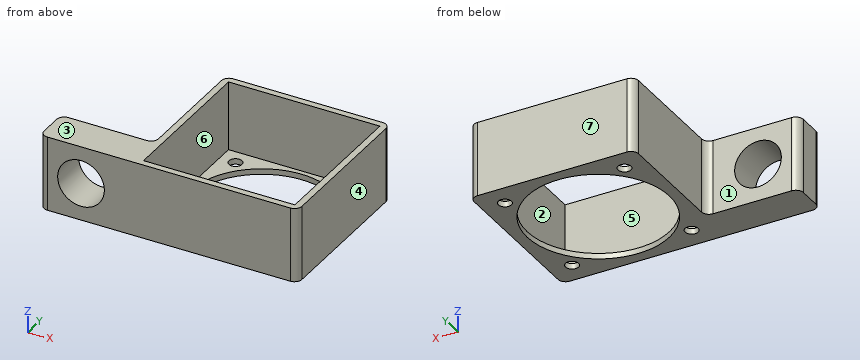
from build123d import *

# Parameters (mm, degrees)
F0_W     = 44
F0_H     = 44
F0_W_2   = 40.5
F0_H_2   = 40.5
F1_DEPTH = 20
F0_R     = 1.75
F0_R_2   = 19
F2_DEPTH = 1.5
F3_W     = 10
F3_H     = 20
F4_DEPTH = 25
F5_R     = 6.25
F6_DEPTH = 10
F7_R     = 2


with BuildPart() as f1:
    # F0 (on Top) → F1 (new body)
    with BuildSketch(Plane.XY):
        Rectangle(F0_W, F0_H)
        Rectangle(F0_W_2, F0_H_2, mode=Mode.SUBTRACT)
    extrude(amount=F1_DEPTH)

    # F0 (on Top) → F2 (join)
    with BuildSketch(Plane.XY):
        Rectangle(F0_W_2, F0_H_2)
        with Locations((-16, -16)):
            Circle(F0_R, mode=Mode.SUBTRACT)
        with Locations((16, -16)):
            Circle(F0_R, mode=Mode.SUBTRACT)
        with Locations((-16, 16)):
            Circle(F0_R, mode=Mode.SUBTRACT)
        Circle(F0_R_2, mode=Mode.SUBTRACT)
        with Locations((16, 16)):
            Circle(F0_R, mode=Mode.SUBTRACT)
    extrude(amount=F2_DEPTH)

    # F3 (on face) → F4 (join)
    with BuildSketch(Plane(origin=(-22, 0, 0), x_dir=(0, -1, 0), z_dir=(-1, 0, 0))):
        with Locations((17, 10)):
            Rectangle(F3_W, F3_H)
    extrude(amount=F4_DEPTH)

    # F5 (on face) → F6 (cut)
    with BuildSketch(Plane(origin=(0, -12, 0), x_dir=(-1, 0, 0), z_dir=(0, 1, 0))):
        with Locations((36, 10)):
            Circle(F5_R)
    extrude(amount=-F6_DEPTH, mode=Mode.SUBTRACT)

    # F7
    f7_edges = [f1.edges().sort_by_distance(p)[0] for p in [
        (-22, -12, 10),
        (-22, 22, 10),
        (22, 22, 10),
        (22, -22, 10),
        (-47, -12, 10),
        (-47, -22, 10),
    ]]
    fillet(f7_edges, radius=F7_R)


solid = f1.part
Read the model definition and answer for the solid it produces. Units are mm, in the model's axes. Face numbers are marked on the shaded views. A direction names the side the tool comes from. Round coordinates to 2 decimals unless told otherwise and drop trailing zeros. Loops run counter-clockwise (first coordinate to the right, second up) from the corner with the lowest first, then second, coordinate; pieces in that order, holes last. Notation, with made-up numbers: (19.5, 39.5) - (51.5, 39.5) arc R28 cw to (51.5, 74.5) - close; hole circle Ø2 at (42, 10). An arc over 180 degrees is marked (long way). One line per question, with ' | ' between items. Start each with the question number.
Q1. Section C-C on y = -16 is taken. Give the vertices of the cut face in (x, z).
Q2. For a pull along Y with two mould halves and no side action, classify the marked faces 4, 5, 6 and 7 as +Y half, -Y half, draft (parallel to the pull), parting line (faces both ways), or undercut.
Q3. Flat-ended cylindrical pins translate along their axes: pin 1 (12 mm diameter, centred on y = 6, z = 6, fed in from -X); pin 2 (5.5 mm diameter, centred on x = -16, y = -16, fed in from +Z); pin 3 (4 mm diameter, centred on x = -14.5, y = 13, fed in from -Z). Find the tip coordinate at first contact, or state that the pin passes through.
Q4. Section A-A on z = 6.25 is taken. Give the vertices of the cut face in (x, y), plus the area to 3 significant figures.
Q5. Section B-B on x = 0 is taken. Give the vertices of the cut face in (y, z), plus the area to 4 significant figures.
Q6. Find the intervals of material crossed by L1, parallel to X at y = 14, z = 3.25; L2, parallel to Y at x = -16, z = 0.65, in increasing order.
Q7. For the marked faces 1, 2 and 3, determine the directions among +Z, -Z, +X, -X, +Y, -Y from which every point of the face is accessible in a straight line to the end or side of a thin tool.
Q8. Section D-D on z = 10 is taken. Give the vertices of the cut face in (x, y).
Established:
1) outline: (-47, 0) - (-17.75, 0) - (-17.75, 1.5) - (-20.25, 1.5) - (-20.25, 20) - (-47, 20) - close; (-14.25, 0) - (-10.25, 0) - (-10.25, 1.5) - (-14.25, 1.5) - close; (10.25, 0) - (14.25, 0) - (14.25, 1.5) - (10.25, 1.5) - close; (17.75, 0) - (22, 0) - (22, 20) - (20.25, 20) - (20.25, 1.5) - (17.75, 1.5) - close; hole circle Ø12.5 at (-36, 10)
2) face 4: draft | face 5: undercut | face 6: undercut | face 7: +Y half
3) pin 1: x = -22 | pin 2: z = 1.5 | pin 3: z = 0
4) outline: (-47, -20) arc R2 ccw to (-45, -22) - (-41, -22) - (-41, -12) - (-45, -12) arc R2 ccw to (-47, -14) - close; (-31, -22) - (20, -22) arc R2 ccw to (22, -20) - (22, 20) arc R2 ccw to (20, 22) - (-20, 22) arc R2 ccw to (-22, 20) - (-22, -10) arc R2 cw to (-24, -12) - (-31, -12) - close; hole (-20.25, -20.25) - (20.25, -20.25) - (20.25, 20.25) - (-20.25, 20.25) - close | area: 442 mm²
5) outline: (-22, 0) - (-19, 0) - (-19, 1.5) - (-20.25, 1.5) - (-20.25, 20) - (-22, 20) - close; (19, 0) - (22, 0) - (22, 20) - (20.25, 20) - (20.25, 1.5) - (19, 1.5) - close | area: 73.75 mm²
6) L1: -22 to -20.25, 20.25 to 22 | L2: -22 to -17.75, -14.25 to -10.25, 10.25 to 14.25, 17.75 to 22
7) face 1: +Z, -Z, -X, +Y | face 2: +Z | face 3: +Z, +X, -X, +Y, -Y
8) outline: (-47, -20) arc R2 ccw to (-45, -22) - (-42.25, -22) - (-42.25, -12) - (-45, -12) arc R2 ccw to (-47, -14) - close; (-29.75, -22) - (20, -22) arc R2 ccw to (22, -20) - (22, 20) arc R2 ccw to (20, 22) - (-20, 22) arc R2 ccw to (-22, 20) - (-22, -10) arc R2 cw to (-24, -12) - (-29.75, -12) - close; hole (-20.25, -20.25) - (20.25, -20.25) - (20.25, 20.25) - (-20.25, 20.25) - close
